from build123d import *

# Parameters (mm, degrees)
BOSS_EXTRUDE1_DEPTH                                  = 101.6
CBORE_FOR_1_4_BINDING_HEAD_MACHINE_SCREW_D           = 6.7564
CBORE_FOR_1_4_BINDING_HEAD_MACHINE_SCREW_CBORE_D     = 14.2875
CBORE_FOR_1_4_BINDING_HEAD_MACHINE_SCREW_CBORE_DEPTH = 4.191


with BuildPart() as part:
    # Sketch1 → Boss-Extrude1 (new body)
    with BuildSketch(Plane.XY):
        Polygon((0, -19.05), (12.7, -6.35), (25.4, -19.05), (25.4, 0), (0, 0), align=None)
    extrude(amount=BOSS_EXTRUDE1_DEPTH)

    # CBORE for 1/4 Binding Head Machine Screw1 (through all)
    with Locations(Plane(origin=(0, 0, 0), x_dir=(1, 0, 0), z_dir=(0, 1, 0))):
        with Locations((12.7, -88.9), (12.7, -12.7)):
            CounterBoreHole(CBORE_FOR_1_4_BINDING_HEAD_MACHINE_SCREW_D / 2, CBORE_FOR_1_4_BINDING_HEAD_MACHINE_SCREW_CBORE_D / 2, CBORE_FOR_1_4_BINDING_HEAD_MACHINE_SCREW_CBORE_DEPTH)


solid = part.part
CAD build for the part. Positions are in the model's coordinates, mm. A direction names the side the tool comes from. Round coordinates to 2 decimals unless told otherwise and drop trailing zeros. Write each loop counter-clockwise with the first axis right and the second up, starting at its lowest first coordinate (ties: lowest second). Pieces come first, ordered by that corner, then holes. Notation, with made-up numbers: M -8,68.5 L 31,68.5 A32 cw 31,96.5 Z; hole C -29.75,18 d10. An arc over 180 degrees is marked long. Put each result on its own line as item: value. Start each with the question number.
1) Saw through at C-C, the plane y = -1.5. Write the cut outline in (x, z), and give its area (3 significant figures).
2) Pin check, flat tips, straight feed: pin 1 Ø8.5 at (x, z) = (12.7, 88.9) entering from -Y; pin 2 Ø4.5 at (x, z) = (15.5, 91.5) entering from +Y; pin 3 Ø1.5 at (x, z) = (6, 25.5) entering from -Y; pin 4 Ø4 at (x, z) = (12.7, 88.9) entering from +Y. Stop position of each tip, or through.
3) Saw through at B-B, the plane z = 12.7. Write the cut outline in (x, y).
4) Saw through at D-D, the plane z = 35.5. Write the cut outline in (x, y).
5) Drill centre lines: probe 1 along Z at (x, y) = (12.7, -1.2); probe 2 along X at (y, z) = (-8.4, 12.7); probe 3 along X at (y, z) = (-0.9, 88.9). Where is each one in solid material? Low to high. Write a range as [from, to].
6) Saw through at A-A, the plane y = -14.25. Write the cut outline in (x, z).
7) 3-axis set-ups, long thin cutter, end or side, ignore diameter. For faces 4 (the cylindrical face through (7.435, -2.066, 7.872)), 5 (the flat face through (13, -5, 101.6)), 6 (the flat face through (18.96, -12.61, 50.09)): which of +Z, -Z, +X, -X, +Y, -Y reach the whole face in a straight line?
8) Pull direction X, two halves, no side cores. Call faces 1 (the flat face through (11, -4.191, 92)), 2 (the flat face through (0, -9, 50)), 3 (the flat face through (13, -5, 0)): pulls with the +X half, pulls with the -X half, needs draft (parallel to the pull), parting line crosses it, or undercut.
Resolved:
1. outline: M 0,0 L 25.4,0 L 25.4,101.6 L 0,101.6 Z; hole C 12.7,12.7 d14.29; hole C 12.7,88.9 d14.29
1. area: 2,260 mm²
2. pin 1: y = -10.6
2. pin 2: y = -4.19
2. pin 3: y = -13.8
2. pin 4: through
3. outline: M 0,-19.05 L 9.32,-9.73 L 9.32,-4.19 L 5.56,-4.19 L 5.56,0 L 0,0 Z; M 16.08,-9.73 L 25.4,-19.05 L 25.4,0 L 19.84,0 L 19.84,-4.19 L 16.08,-4.19 Z
4. outline: M 0,-19.05 L 12.7,-6.35 L 25.4,-19.05 L 25.4,0 L 0,0 Z
5. probe 1: [0, 5.56], [19.84, 81.76], [96.04, 101.6]
5. probe 2: [0, 9.32], [16.08, 25.4]
5. probe 3: [0, 5.56], [19.84, 25.4]
6. outline: M 0,0 L 4.8,0 L 4.8,101.6 L 0,101.6 Z; M 20.6,0 L 25.4,0 L 25.4,101.6 L 20.6,101.6 Z
7. face 4: +Y
7. face 5: +Z, +X, -X, +Y, -Y
7. face 6: +Z, -Z, -Y
8. face 1: undercut
8. face 2: pulls with the -X half
8. face 3: needs draft
